Read the model definition and answer for the solid it produces. Units are mm, in the model's axes. Face numbers are marked on the shaded views. A direction names the side the tool comes from. Give positions to 0.01 mm unless a question says otherwise; leave off trailing zeros. Order: outer loops, then holes, each group sorted by start corner. A loop starts at its lowest first (then second) coordinate and runs counter-clockwise, first axis right, second up.
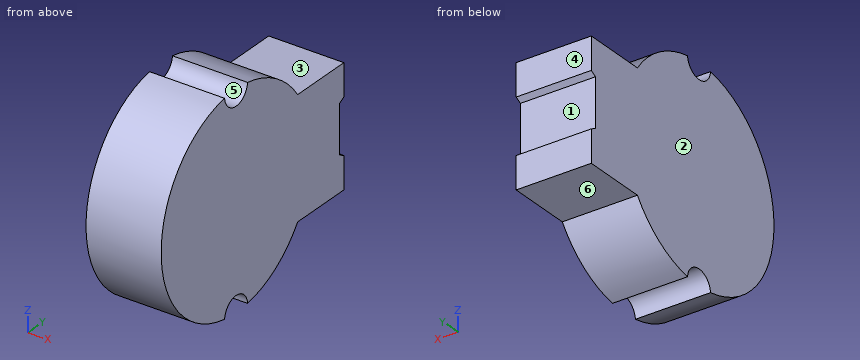
```python
from build123d import *

# Parameters (mm, degrees)
BOSS_EXTRUDE1_DEPTH = 14


with BuildPart() as part:
    # Sketch1 → Boss-Extrude1 (new body)
    with BuildSketch(Plane(origin=(0, 0, 0), x_dir=(0, 0, -1), z_dir=(1, 0, 0))):
        with BuildLine():
            Line((-4.5, 22.673860989), (4.5, 22.673860989))
            Line((4.5, 22.673860989), (5.1, 23.773860989))
            Line((5.1, 23.773860989), (11.1, 23.773860989))
            Line((11.1, 23.773860989), (11.1, 11.75860607))
            ThreePointArc((11.1, 11.75860607), (16.525488971, 6.077864194), (19.269230769, -1.282749897))
            ThreePointArc((19.269230769, -1.282749897), (16.5, -4.273860989), (19.269230769, -7.26497208))
            ThreePointArc((19.269230769, -7.26497208), (0, -23.773860989), (-19.269230769, -7.26497208))
            ThreePointArc((-19.269230769, -7.26497208), (-16.5, -4.273860989), (-19.269230769, -1.282749897))
            ThreePointArc((-19.269230769, -1.282749897), (-16.525488971, 6.077864194), (-11.1, 11.75860607))
            Line((-11.1, 11.75860607), (-11.1, 23.773860989))
            Line((-11.1, 23.773860989), (-5.1, 23.773860989))
            Line((-5.1, 23.773860989), (-4.5, 22.673860989))
        make_face()
    extrude(amount=BOSS_EXTRUDE1_DEPTH)


solid = part.part
```
1) The part is cut by section A-A on x = 3.25. Determine the outline of the cut face in (y, z).
Final values:
outline: (-7.26, -19.27) arc R3 cw to (-1.28, -19.27) arc R19.5 ccw to (11.76, -11.1) - (23.77, -11.1) - (23.77, -5.1) - (22.67, -4.5) - (22.67, 4.5) - (23.77, 5.1) - (23.77, 11.1) - (11.76, 11.1) arc R19.5 ccw to (-1.28, 19.27) arc R3 cw to (-7.26, 19.27) arc R19.5 ccw to start
2) The part is cut by section C-C on y = -6.5. Determine the outline of the cut face in (x, z), and give its area (3 significant figures).
Final values:
outline: (0, -17.49) - (14, -17.49) - (14, 17.49) - (0, 17.49) - close
area: 490 mm2
3) Consider L1, parallel to Z at x = 9, y = 13; L2, parallel to Y at x = 1, z = 17.5; L3, parallel to Z at x = 8.75, y = -4.5. Determine where each line is inside the solid, lowest interval first.
Final values:
L1: z = -11.1 to 11.1
L2: y = -12.88 to -6.51, -2.04 to 4.33
L3: z = -16.51 to 16.51
4) Given pin 1 (2.5 mm diameter, centred on x = 7.5, z = -1, fed in from +Y); pin 2 (3 mm diameter, centred on x = 12.5, y = -9.5, fed in from +Z); pin 3 (3 mm diameter, centred on x = 6.5, y = -14.5, fed in from +Z), each flat-ended and moving along its own axis, determine where each tip first touches the part or whether it passes through.
Final values:
pin 1: stops at y = 22.67
pin 2: stops at z = 19.14
pin 3: stops at z = 17.44
5) For a pull along Y with two mould halves and no side action, classify the marked faces 4, 5 and 6 as released by +Y, released by -Y, zero draft, split by the parting line, or undercut.
Final values:
face 4: released by +Y
face 5: undercut
face 6: zero draft
6) The part is cut by section B-B on z = -1.5. Determine the outline of the cut face in (x, y), and give its area (3 significant figures).
Final values:
outline: (0, -23.72) - (14, -23.72) - (14, 22.67) - (0, 22.67) - close
area: 649 mm2
7) A tool of negligible diameter and unlimited length cuts with its end or side. For the marked faces 1, 2 and 3, from which of +Z, -Z, +X, -X, +Y, -Y can it reach the whole face along a straight path? Write none if from no direction.
Final values:
face 1: +X, -X, +Y
face 2: +Z, -Z, -X, +Y, -Y
face 3: +Z, +X, -X, +Y
